from build123d import *

# Parameters (mm, degrees)
SKETCH_2_W          = 35
SKETCH_2_H          = 58
EXTRUDE_1_DEPTH     = 2.5
SKETCH_4_W          = 7.5
SKETCH_4_H          = 3
CUT_EXTRUDE_1_DEPTH = 3.5
CUT_EXTRUDE_2_DEPTH = 3.5
SKETCH_7_R          = 2.5
SKETCH_7_W          = 15
SKETCH_7_H          = 17
CUT_EXTRUDE_3_DEPTH = 3.5
FILLET_1_R          = 1


with BuildPart() as part:
    # 草图2 → 凸台-拉伸1 (new body)
    with BuildSketch(Plane(origin=(0, 0, 0), x_dir=(0, 0, -1), z_dir=(1, 0, 0))):
        Rectangle(SKETCH_2_W, SKETCH_2_H)
    extrude(amount=EXTRUDE_1_DEPTH)

    # 草图4 → 切除-拉伸1 (cut, through all)
    with BuildSketch(Plane.ZY):
        with Locations((-8.95, 24.5)):
            Rectangle(SKETCH_4_W, SKETCH_4_H)
        with Locations((10.95, 24.5)):
            Rectangle(SKETCH_4_W, SKETCH_4_H)
        with Locations((-8.95, -24.5)):
            Rectangle(SKETCH_4_W, SKETCH_4_H)
        with Locations((10.95, -24.5)):
            Rectangle(SKETCH_4_W, SKETCH_4_H)
    extrude(amount=-CUT_EXTRUDE_1_DEPTH, mode=Mode.SUBTRACT)

    # 草图5 → 切除-拉伸2 (cut, through all)
    with BuildSketch(Plane.ZY):
        with BuildLine():
            Line((-17.5, 29), (-17.5, 26.000000007))
            ThreePointArc((-17.5, 26.000000007), (-16.621320341, 28.121320346), (-14.5, 29))
            Line((-14.5, 29), (-17.5, 29))
        make_face()
        with BuildLine():
            Line((-14.5, 0), (-14.5, 23))
            ThreePointArc((-14.5, 23), (-16.621320346, 23.878679659), (-17.5, 26.000000007))
            Line((-17.5, 26.000000007), (-17.5, 0))
            Line((-17.5, 0), (-14.5, 0))
        make_face()
        with BuildLine():
            Line((-14.5, -23), (-14.5, 0))
            Line((-14.5, 0), (-17.5, 0))
            Line((-17.5, 0), (-17.5, -26))
            ThreePointArc((-17.5, -26), (-16.621320344, -23.878679656), (-14.5, -23))
        make_face()
        with BuildLine():
            ThreePointArc((-14.5, -29), (-16.621320344, -28.121320344), (-17.5, -26))
            Line((-17.5, -26), (-17.5, -29))
            Line((-17.5, -29), (-14.5, -29))
        make_face()
    extrude(amount=-CUT_EXTRUDE_2_DEPTH, mode=Mode.SUBTRACT)

    # 草图7 → 切除-拉伸3 (cut, through all)
    with BuildSketch(Plane.ZY):
        with Locations((7, 9.7)):
            Circle(SKETCH_7_R)
        with Locations((4.5, -8)):
            Rectangle(SKETCH_7_W, SKETCH_7_H)
    extrude(amount=-CUT_EXTRUDE_3_DEPTH, mode=Mode.SUBTRACT)

    # 圆角1
    fillet_1_edges = [part.edges().sort_by_distance(p)[0] for p in [
        (1.25, -29, 17.5),
        (1.25, 29, 17.5),
    ]]
    fillet(fillet_1_edges, radius=FILLET_1_R)


solid = part.part
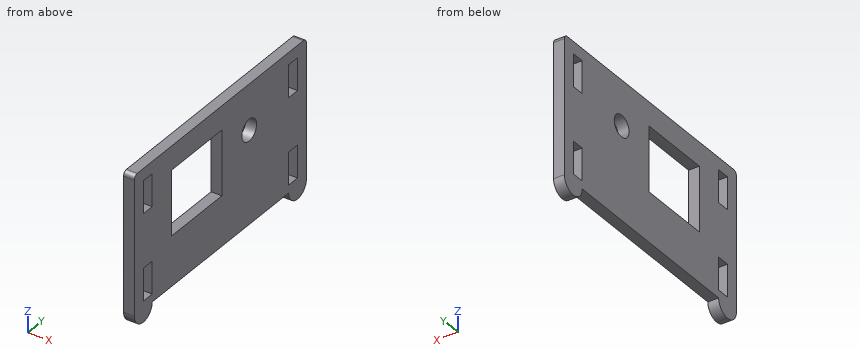
Read the model definition and answer for the solid it produces. Units are mm, in the model's axes. Round coordinates to 2 decimals unless told otherwise and drop trailing zeros. Write each loop counter-clockwise with the first axis right and the second up, starting at its lowest first coordinate (ties: lowest second). Pieces come first, ordered by that corner, then holes.
1. The part is cut by section C-C, the plane z = -8.5. Determine the outline of the cut face in (x, y).
2. The part is cut by section A-A, the plane x = 1.75. State how many separate pieces and enclosed holes the cut face has, then the cut area to 3 significant figures.
3. The part is cut by section D-D, the plane z = 10.5. Determine the outline of the cut face in (x, y).
4. Given pin 1 Ø8 at (y, z) = (9.7, 7) entering from -X; pin 2 Ø1.5 at (x, y) = (0.5, 7.5) entering from -Z, each flat-ended and moving along its own axis, determine where each tip first touches the part or whether it passes through.
5. The part is cut by section B-B, the plane y = -8. Determine the outline of the cut face in (x, z), then the cut area to 3 significant figures.
6. Straight lines are drawn through the part: L1, parallel to Y at x = 1.7, z = 7; L2, parallel to Y at x = 0.7, z = 12.5; L3, parallel to Y at x = 2.3, z = 10. For each, find the intervals that lie inside material, in ascending order.
Values:
1. outline: (0, -29) - (2.5, -29) - (2.5, -26) - (0, -26) - close; (0, -23) - (2.5, -23) - (2.5, 23) - (0, 23) - close; (0, 26) - (2.5, 26) - (2.5, 29) - (0, 29) - close
2. separate pieces: 1
2. enclosed holes: 6
2. area: 1,520 mm2
3. outline: (0, -29) - (2.5, -29) - (2.5, -26) - (0, -26) - close; (0, -23) - (2.5, -23) - (2.5, -16.5) - (0, -16.5) - close; (0, 0.5) - (2.5, 0.5) - (2.5, 23) - (0, 23) - close; (0, 26) - (2.5, 26) - (2.5, 29) - (0, 29) - close
4. pin 1: stops at x = 0
4. pin 2: stops at z = -14.5
5. outline: (0, -14.5) - (2.5, -14.5) - (2.5, -3) - (0, -3) - close; (0, 12) - (2.5, 12) - (2.5, 17.5) - (0, 17.5) - close
5. area: 42.5 mm2
6. L1: y = -29 to -16.5, 0.5 to 7.2, 12.2 to 29
6. L2: y = -29 to -26, -23 to 23, 26 to 29
6. L3: y = -29 to -26, -23 to -16.5, 0.5 to 23, 26 to 29
